The listing builds one solid part. Answer for the finished solid, in the listing's coordinates (mm). Face numbers are marked on the shaded views. A direction names the side the tool comes from. Round coordinates to 2 decimals unless told otherwise and drop trailing zeros. Order: outer loops, then holes, each group sorted by start corner. A loop starts at its lowest first (then second) coordinate and runs counter-clockwise, first axis right, second up. Notation, with made-up numbers: (42.25, 48.5) -> (54.25, 48.5) arc R27 cw to (54.25, 83.5) -> close; hole circle Ø11 at (77.25, -33.75). An arc over 180 degrees is marked (long way). Return JSON: item names as keys, results as strings. Group by question number.
(1) The part is cut by section C-C (x = 0). Determine the outline of the cut face in (y, z), plus the area to 3 significant figures.
(2) The part is cut by section D-D (y = 0). Determine the outline of the cut face in (x, z).
(3) The part is cut by section A-A (x = 262). Determine the outline of the cut face in (y, z), plus the area to 3 significant figures.
(4) Consider line 1 (Z direction, x = 209, y = -111); line 2 (Z direction, x = 15, y = -229.5); line 3 (X direction, y = -260, z = -1205). Determine where each line is inside the solid, lowest interval first. Write a range as [from, to].
(5) Determine the mould class of the marked faces 5, 6 and 7 for opening direction Z: +Z half, -Z half, draft (parallel to the pull), parting line (faces both ways), or undercut.
(6) Which of the six approach directions +Z, -Z, +X, -X, +Y, -Y give full straight-line access (tool end or side, diameter ignored) to the marked faces 1, 2, 3 and 4?
(7) The part is cut by section B-B (y = 91). Determine the outline of the cut face in (x, z).
(8) Each of these flat-tipped pins is pushed along its axis until it touches: pin 1 (3 mm diameter, centred on x = 220, z = -964.5, fed in from -Y); pin 2 (3 mm diameter, centred on x = -24.5, z = -1390, fed in from -Y); pin 3 (1 mm diameter, centred on x = -61.5, z = -274.5, fed in from +Y). Where does it stop, or does it pass through?
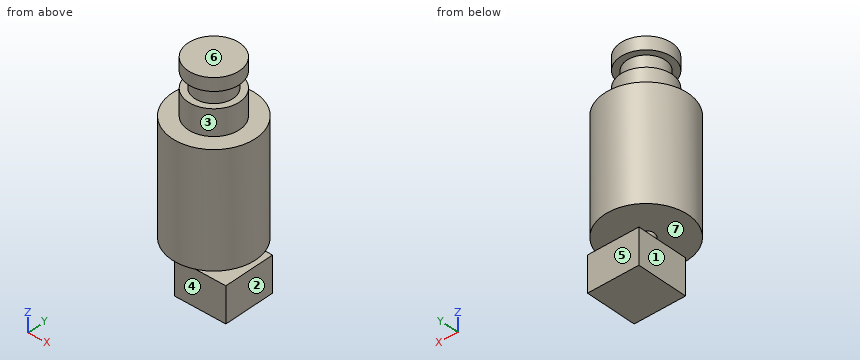
from build123d import *

# Parameters (mm, degrees)
F0_R      = 203.2
F1_DEPTH  = 101.6
F2_R      = 152.4
F3_DEPTH  = 127
F4_R      = 203.2
F5_DEPTH  = 203.2
F6_R      = 330.2
F7_DEPTH  = 889
F8_R      = 63.5
F9_DEPTH  = 101.6
F10_W     = 406.4
F10_H     = 406.4
F10_R     = 63.5
F11_DEPTH = 279.4


with BuildPart() as f1:
    # F0 (on Top) → F1 (new body)
    with BuildSketch(Plane.XY):
        Circle(F0_R)
    extrude(amount=F1_DEPTH)

    # F2 (on face) → F3 (join)
    with BuildSketch(Plane(origin=(0, 0, 0), x_dir=(1, 0, 0), z_dir=(0, 0, -1))):
        Circle(F2_R)
    extrude(amount=F3_DEPTH)

    # F4 (on face) → F5 (join)
    with BuildSketch(Plane(origin=(0, 0, -127), x_dir=(1, 0, 0), z_dir=(0, 0, -1))):
        Circle(F4_R)
    extrude(amount=F5_DEPTH)

    # F6 (on face) → F7 (join)
    with BuildSketch(Plane(origin=(0, 0, -330.2), x_dir=(1, 0, 0), z_dir=(0, 0, -1))):
        Circle(F6_R)
    extrude(amount=F7_DEPTH)

    # F8 (on face) → F9 (join)
    with BuildSketch(Plane(origin=(0, 0, -1219.2), x_dir=(1, 0, 0), z_dir=(0, 0, -1))):
        Circle(F8_R)
    extrude(amount=F9_DEPTH)

    # F10 (on face) → F11 (join)
    with BuildSketch(Plane(origin=(0, 0, -1320.8), x_dir=(1, 0, 0), z_dir=(0, 0, -1))):
        with Locations((76.2, 0)):
            Rectangle(F10_W, F10_H)
        Circle(F10_R, mode=Mode.SUBTRACT)
        Circle(F10_R)
    extrude(amount=F11_DEPTH)


solid = f1.part
Answer below:
{
 "1": {"outline": "(-330.2, -1219.2) -> (-63.5, -1219.2) -> (-63.5, -1320.8) -> (-203.2, -1320.8) -> (-203.2, -1600.2) -> (203.2, -1600.2) -> (203.2, -1320.8) -> (63.5, -1320.8) -> (63.5, -1219.2) -> (330.2, -1219.2) -> (330.2, -330.2) -> (203.2, -330.2) -> (203.2, -127) -> (152.4, -127) -> (152.4, 0) -> (203.2, 0) -> (203.2, 101.6) -> (-203.2, 101.6) -> (-203.2, 0) -> (-152.4, 0) -> (-152.4, -127) -> (-203.2, -127) -> (-203.2, -330.2) -> (-330.2, -330.2) -> close", "area": "876,000 mm²"},
 "2": {"outline": "(-330.2, -1219.2) -> (-63.5, -1219.2) -> (-63.5, -1320.8) -> (-127, -1320.8) -> (-127, -1600.2) -> (279.4, -1600.2) -> (279.4, -1320.8) -> (63.5, -1320.8) -> (63.5, -1219.2) -> (330.2, -1219.2) -> (330.2, -330.2) -> (203.2, -330.2) -> (203.2, -127) -> (152.4, -127) -> (152.4, 0) -> (203.2, 0) -> (203.2, 101.6) -> (-203.2, 101.6) -> (-203.2, 0) -> (-152.4, 0) -> (-152.4, -127) -> (-203.2, -127) -> (-203.2, -330.2) -> (-330.2, -330.2) -> close"},
 "3": {"outline": "(-203.2, -1600.2) -> (203.2, -1600.2) -> (203.2, -1320.8) -> (-203.2, -1320.8) -> close; (-200.97, -1219.2) -> (200.97, -1219.2) -> (200.97, -330.2) -> (-200.97, -330.2) -> close", "area": "471,000 mm²"},
 "4": {"line 1": "z = [-1600.2, -1320.8], [-1219.2, -330.2]", "line 2": "z = [-1219.2, -330.2]", "line 3": "x = [-203.55, 203.55]"},
 "5": {"face 5": "draft", "face 6": "+Z half", "face 7": "undercut"},
 "6": {"face 1": "-Z, -X, +Y, -Y", "face 2": "-Z, +X, +Y, -Y", "face 3": "+Z", "face 4": "-Z, +X, -X, -Y"},
 "7": {"outline": "(-317.41, -1219.2) -> (317.41, -1219.2) -> (317.41, -330.2) -> (181.68, -330.2) -> (181.68, -127) -> (122.25, -127) -> (122.25, 0) -> (181.68, 0) -> (181.68, 101.6) -> (-181.68, 101.6) -> (-181.68, 0) -> (-122.25, 0) -> (-122.25, -127) -> (-181.68, -127) -> (-181.68, -330.2) -> (-317.41, -330.2) -> close; (-127, -1600.2) -> (279.4, -1600.2) -> (279.4, -1320.8) -> (-127, -1320.8) -> close"},
 "8": {"pin 1": "stops at y = -247.57", "pin 2": "stops at y = -203.2", "pin 3": "stops at y = 193.83"}
}
